Model file for the job. Use its own axes, mm. Give positions to 0.01 mm unless a question says otherwise; leave off trailing zeros. Write each loop counter-clockwise with the first axis right and the second up, starting at its lowest first coordinate (ties: lowest second). Pieces come first, ordered by that corner, then holes.
Autodesk Inventor part; units mm, degrees
ref_plane "YZ Plane" through (0, 0, 0) normal (1, 0, 0) x (0, 1, 0)
ref_plane "XZ Plane" through (0, 0, 0) normal (0, 1, 0) x (-1, 0, 0)
ref_plane "XY Plane" through (0, 0, 0) normal (0, 0, 1) x (1, 0, 0)
sketch "Sketch1" plane through (0, 0, 0) normal (0, 0, 1) x (1, 0, 0)
  arc A0 (0.1634, -151.6592) -> (162.48, -141.1714) centre (0.1634, 1109.6463) ccw
  arc A1 (0.1634, -136.6592) -> (171.9535, -124.7627) centre (0.1634, 1109.6463) ccw
  line L0 (171.9535, -124.7627) -> (162.48, -141.1714)
  line L1 (171.9535, -124.7627) -> (190.9007, -124.7627) construction
  line L2 (0.1634, -151.6592) -> (0.1634, -124.7627)
  arc A2 (-162.1531, -141.1714) -> (0.1634, -151.6592) centre (0.1634, 1109.6463) ccw
  arc A3 (-171.6266, -124.7627) -> (0.1634, -136.6592) centre (0.1634, 1109.6463) ccw
  line L3 (-171.6266, -124.7627) -> (-162.1531, -141.1714)
  point P0 (0, 0)
  dimension "d0" = 15
  dimension "d1" = 120
extrude "Extrusion1" add sketch "Sketch1" along normal blind 30
fillet "Fillet1" radius 3 12 edges at (-85.9373, -133.6816, 30) (81.4909, -149.0346, 30) (167.2167, -132.9671, 30) (171.9535, -124.7627, 15) (162.48, -141.1714, 15) (167.2167, -132.9671, 0) (-166.8899, -132.9671, 30) (-171.6266, -124.7627, 15) (86.2642, -133.6816, 0) (81.4909, -149.0346, 0) (-162.1531, -141.1714, 15) (-166.8899, -132.9671, 0)
sketch "Sketch2" plane through (0, 0, 0) normal (0, 1, 0) x (-1, 0, 0)
  line L0 (0, 0) -> (0, 15)
  circle A0 centre (0, 15) radius 5
  dimension "d5" = 15
  dimension "d6" = 10
extrude "Extrusion2" cut sketch "Sketch2" against normal blind 300
properties part number "LEAF 6" material "Steel, Carbon"
1. Probe probe 1 along Z at (x, y) = (0, -139.75); probe 2 along Z at (x, y) = (113, -134); probe 3 along X at (y, z) = (-140, 15). List the from-to ranges inside material, lowest first.
Calculated:
probe 1: z = 0 to 10, 20 to 30
probe 2: z = 0.05 to 29.95
probe 3: x = -162.83 to -5, 5 to 163.15
2. Pin check, flat tips, straight feed: P1, Ø4, axis at y = -137, z = 12.5, coming from the -X side; P2, Ø8, axis at y = -134.5, z = 26.5, coming from the -X side; P3, Ø10, axis at y = -137.5, z = 18.5, coming from the +X side; P4, Ø6, axis at x = 0, z = 15, coming from the +Y side. Stop position of each tip, or through.
Calculated:
P1: stops at x = -165.72
P2: stops at x = -168.31
P3: stops at x = 167.49
P4: passes through
3. Pull direction X, two halves, no side cores. Call faces 1 (the cylindrical face through (165.277, -134.616, 29.098)), 2 (the cylindrical face through (-81.726, -133.966, 14.832)), 3 (the cylindrical face through (84.38, -133.81, 14.83)), 4 (the flat face through (-2, -141, 30)): +X half, -X half, draft (parallel to the pull), parting line (faces both ways), or undercut.
Calculated:
face 1: +X half
face 2: undercut
face 3: undercut
face 4: draft
4. Slice it at A-A, the plane z = 23.25. Write the cut outline in (x, y).
Calculated:
outline: (-168.57, -130.06) - (-162.9, -139.89) arc R3 ccw to (-160.68, -141.36) arc R1261.31 ccw to (0.16, -151.66) arc R1261.31 ccw to (161.01, -141.36) arc R3 ccw to (163.22, -139.89) - (168.89, -130.06) arc R3 ccw to (165.9, -125.59) arc R1246.31 cw to (0.16, -136.66) arc R1246.31 cw to (-165.57, -125.59) arc R3 ccw to start
